from build123d import *

# Parameters (mm, degrees)
BASPROSKE_W        = 10
BASPROSKE_H        = 11
TOOTHCUT_DEPTH     = 19.493242009
TEETHCUTS_COUNT    = 20
TEETHCUTS_ANGLE    = 342
BORSKE_R           = 0.75
BORE_DEPTH         = 50.0000508
CUT_EXTRUDE1_DEPTH = 4.5
SKETCH2_R          = 1.3
CUT_EXTRUDE2_DEPTH = 10
SKETCH3_R          = 3
CUT_EXTRUDE3_DEPTH = 0.5


with BuildPart() as part:
    # BasProSke → Base-Revolve (revolve)
    with BuildSketch(Plane(origin=(0, 0, 0), x_dir=(1, 0, 0), z_dir=(0, 1, 0)), mode=Mode.PRIVATE) as base_revolve_sk:
        with Locations((5, 5.5)):
            Rectangle(BASPROSKE_W, BASPROSKE_H)
    revolve(base_revolve_sk.sketch.rotate(Axis((-10, 0, 0), (1, 0, 0)), 180), axis=Axis((-10, 0, 0), (1, 0, 0)))

    # TooCutSke → ToothCut (cut, through all)
    with BuildSketch(Plane(origin=(0, 0, 0), x_dir=(0, 0, -1), z_dir=(1, 0, 0))):
        with BuildLine():
            ThreePointArc((0.589353609, 8.729127295), (0, 8.749), (-0.589353609, 8.729127295))
            ThreePointArc((-0.589353609, 8.729127295), (-0.82475631, 9.893403384), (-1.391689312, 10.937213814))
            ThreePointArc((-1.391689312, 10.937213814), (0, 11.0254), (1.391689312, 10.937213814))
            ThreePointArc((1.391689312, 10.937213814), (0.82475631, 9.893403384), (0.589353609, 8.729127295))
        make_face()
    toothcut = extrude(amount=TOOTHCUT_DEPTH, mode=Mode.SUBTRACT)

    # TeethCuts: ToothCut ×20 about axis
    teethcuts_axis = Axis((-10, 0, 0), (1, 0, 0))
    for i in range(1, TEETHCUTS_COUNT):
        add(toothcut.rotate(teethcuts_axis, i * TEETHCUTS_ANGLE / (TEETHCUTS_COUNT - 1)), mode=Mode.SUBTRACT)

    # BorSke → Bore (cut, symmetric)
    with BuildSketch(Plane(origin=(0, 0, 0), x_dir=(0, 0, -1), z_dir=(1, 0, 0))):
        with Locations(Location((0, 0, 0), (0, 0, 180))):
            Circle(BORSKE_R)
    extrude(amount=BORE_DEPTH, both=True, mode=Mode.SUBTRACT)

    # Sketch1 → Cut-Extrude1 (cut)
    with BuildSketch(Plane(origin=(10, 0, 0), x_dir=(0, 0, -1), z_dir=(1, 0, 0))):
        with BuildLine():
            Line((0, 3.6), (6.2, 3.6))
            Line((6.2, 3.6), (6.2, -3.6))
            Line((6.2, -3.6), (0, -3.6))
            ThreePointArc((0, -3.6), (-3.6, 0), (0, 3.6))
        make_face()
    extrude(amount=-CUT_EXTRUDE1_DEPTH, mode=Mode.SUBTRACT)

    # Sketch2 → Cut-Extrude2 (cut)
    with BuildSketch(Plane.ZY):
        Circle(SKETCH2_R)
    extrude(amount=-CUT_EXTRUDE2_DEPTH, mode=Mode.SUBTRACT)

    # Sketch3 → Cut-Extrude3 (cut)
    with BuildSketch(Plane.ZY):
        Circle(SKETCH3_R)
    extrude(amount=-CUT_EXTRUDE3_DEPTH, mode=Mode.SUBTRACT)


solid = part.part
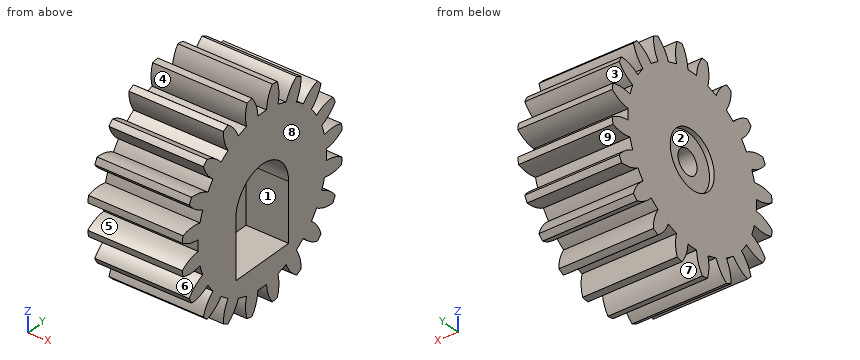
Geometry: final body of the model. Coordinates: model frame, mm. Face numbers are marked on the shaded views. A direction names the side the tool comes from. Coordinates: 2 decimals unless noted, no trailing zeros. Order: outer loops, then holes, each group sorted by start corner. A loop starts at its lowest first (then second) coordinate and runs counter-clockwise, first axis right, second up.
(1) Draft query along Z for the marked faces 6, 7, 8 and 9. Return one class per face: pulls with the +Z half, pulls with the -Z half, needs draft (parallel to the pull), parting line crosses it, or undercut.
(2) Section query B-B (z = -1). Return the cut outline in (x, y).
(3) First-contact query: pin 1 (3 mm diameter, centred on y = -1, z = -0.5, fed in from -X); pin 2 (5 mm diameter, centred on x = 2, y = 8, fed in from -Z); pin 3 (1.3 mm diameter, centred on x = 7, z = -4, fed in from +Y). Flat tips, straight axial feed; report the tip coordinate or a pass-through.
(4) Material intervals for probe 1 along Y at (x, z) = (2.2, 0); probe 2 along Y at (x, z) = (7, 9.25); probe 3 along Y at (x, z) = (1, 7), sorted ascending.
(5) Section query A-A (y = 0). Return the cut outline in (x, z).
(6) Access query for the marked faces 1, 2, 3, 4 and 5. Directions: +Z, -Z, +X, -X, +Y, -Y. A direction counts if a zero-diameter tool reaches every point of the face in a straight line with its end or side. Return the directions, or none.
(7) Section query C-C (z = -3.75). Return the cut outline in (x, y).
Solution:
1. face 6: undercut
1. face 7: pulls with the -Z half
1. face 8: needs draft
1. face 9: undercut
2. outline: (0, -10.3) - (10, -10.3) - (10, -3.6) - (5.5, -3.6) - (5.5, -0.83) - (0.5, -0.83) - (0.5, -2.83) - (0, -2.83) - close; (0, 2.83) - (0.5, 2.83) - (0.5, 0.83) - (5.5, 0.83) - (5.5, 3.6) - (10, 3.6) - (10, 10.3) - (0, 10.3) - close
3. pin 1: stops at x = 0.5
3. pin 2: stops at z = -8.02
3. pin 3: stops at y = 9.93
4. probe 1: y = -8.75 to -1.3, 1.3 to 8.75
4. probe 2: y = -5.29 to -3.92, -2.27 to -0.65, 0.65 to 2.27, 3.92 to 5.29
4. probe 3: y = -7.82 to -5.86, -5.25 to 5.25, 5.86 to 7.82
5. outline: (0, -8.75) - (10, -8.75) - (10, -6.2) - (5.5, -6.2) - (5.5, -1.3) - (0.5, -1.3) - (0.5, -3) - (0, -3) - close; (0, 3) - (0.5, 3) - (0.5, 1.3) - (5.5, 1.3) - (5.5, 3.6) - (10, 3.6) - (10, 8.75) - (0, 8.75) - close
6. face 1: +X
6. face 2: -X
6. face 3: +X, -X, +Y
6. face 4: +X, -X
6. face 5: +X, -X, -Y
7. outline: (0, -9.03) - (10, -9.03) - (10, -3.6) - (5.5, -3.6) - (5.5, 3.6) - (10, 3.6) - (10, 9.03) - (0, 9.03) - close
